Read the model definition and answer for the solid it produces. Units are mm, in the model's axes. Face numbers are marked on the shaded views. A direction names the side the tool comes from. Coordinates: 2 decimals unless noted, no trailing zeros. Write each loop counter-clockwise with the first axis right and the second up, starting at its lowest first coordinate (ties: lowest second). Pieces come first, ordered by that corner, then holes. Notation, with made-up numbers: (-37.5, -7) -> (-1.5, -7) arc R16 ccw to (-1.5, -3) -> close; hole circle Ø3 at (45, -13.75). An arc over 180 degrees is marked (long way). One line per item, written item: value. Start each with the question number.
1. Find section B-B, the plane z = 1. Write down the section's boundary in (x, y).
2. Consider line 1 along Y through (x, z) = (-8.5, 7); line 2 along Y through (x, z) = (6.5, 7.25); line 3 along X through (y, z) = (12.5, 9). Determine where each line is inside the solid, lowest interval first.
3. Given P1, Ø4, axis at y = 8.5, z = 7, coming from the -X side; P2, Ø1, axis at x = 8, z = 6.5, coming from the +Y side; P3, Ø1, axis at x = 4, z = 2.5, coming from the +Y side, each flat-ended and moving along its own axis, determine where each tip first touches the part or whether it passes through.
4. For the marked faces 1 and 2, determine the directions among +Z, -Z, +X, -X, +Y, -Y from which every point of the face is accessible in a straight line to the end or side of a thin tool.
5. Find section A-A, the plane x = 0.75. Write down the section's boundary in (y, z).
6. Find section C-C, the plane y = 9.5. Write down the section's boundary in (x, z), and give its area (3 significant figures).
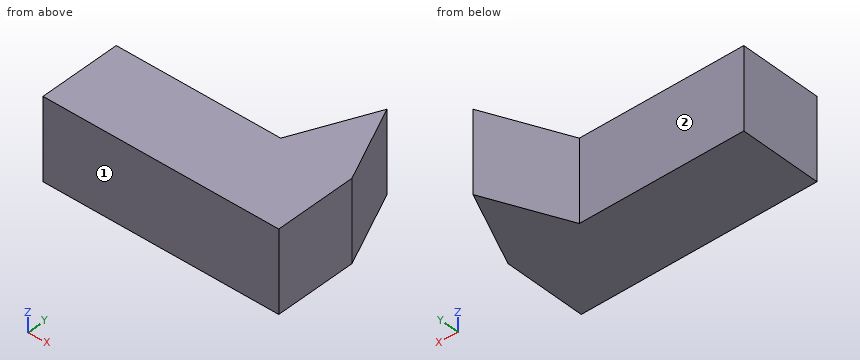
```python
from build123d import *

# Parameters (mm, degrees)
F1_DEPTH = 10


with BuildPart() as f1:
    # F0 (on Top) → F1 (new body)
    with BuildSketch(Plane.XY):
        Polygon((5.733538, 5), (-14.5, 5), (-14.5, -5), (14.5, -5), (14.5, 5), align=None)
        Polygon((10.116769, 14.651284), (5.733538, 5), (14.5, 5), align=None)
    extrude(amount=F1_DEPTH)


solid = f1.part
```
Answer block:
1. outline: (-14.5, -5) -> (14.5, -5) -> (14.5, 5) -> (10.12, 14.65) -> (5.73, 5) -> (-14.5, 5) -> close
2. line 1: y = -5 to 5
2. line 2: y = -5 to 6.69
2. line 3: x = 9.14 to 11.09
3. P1: stops at x = 6.41
3. P2: stops at y = 11.09
3. P3: stops at y = 5
4. face 1: +Z, -Z, +X, -X, -Y
4. face 2: +Z, -Z, -X, +Y
5. outline: (-5, 0) -> (5, 0) -> (5, 10) -> (-5, 10) -> close
6. outline: (7.78, 0) -> (12.46, 0) -> (12.46, 10) -> (7.78, 10) -> close
6. area: 46.8 mm2
